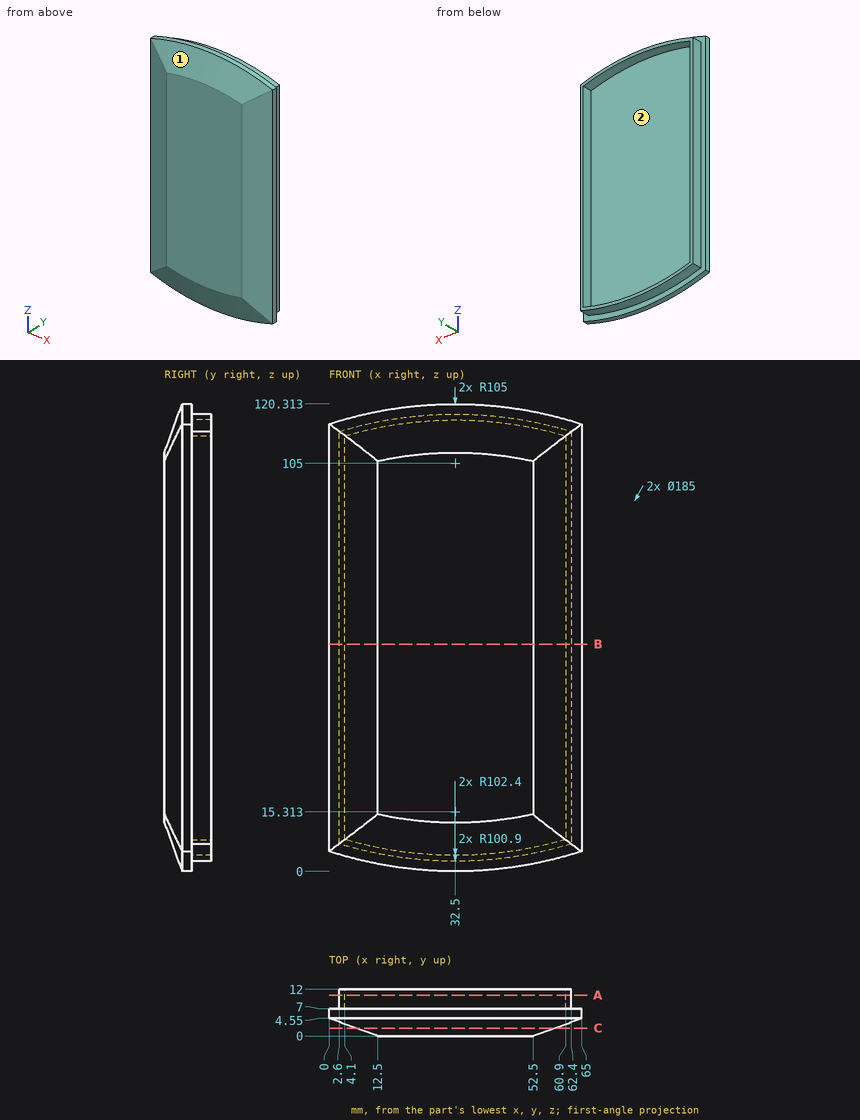
Job drawing, mm, ordinate dimensions from the low corner. One solid piece. A direction names the side the tool comes from. Round coordinates to 2 decimals unless told otherwise and drop trailing zeros. Loops run counter-clockwise (first coordinate to the right, second up) from the corner with the lowest first, then second, coordinate; pieces in that order, holes last.
Item 1: Drill centre lines: line 1 (X direction, y = 8, z = 104); line 2 (Z direction, x = 11.5, y = 10.5); line 3 (Z direction, x = 26.5, y = 8) (1 decimal). Where is each one in solid material? Low to high.
Item 2: Cut at C-C, the plane y = 2. Give the cut face in (x, z) (1 decimal), then the cut area to 3 significant figures.
Item 3: 3-axis set-ups, long thin cutter, end or side, ignore diameter. For the marked faces 1 and 2: which of +Z, -Z, +X, -X, +Y, -Y reach the whole face in a straight line?
Item 4: Cut at A-A, the plane y = 10.5. Give the cut face in (x, z).
Item 5: Drop flat-ended pins along their axis: P1, Ø6, axis at x = 50, y = 10.5, coming from the +Z side; P2, Ø2, axis at y = 4, z = 38.5, coming from the -X side; P3, Ø2.5, axis at y = 8.5, z = 43.5, coming from the -X side; P4, Ø5, axis at x = 52.5, y = 3, coming from the +Z side. Give the stop position or say it passes through.
Item 6: Cut at B-B, the plane z = 58.5. Give the cut face in (x, y).
A:
1. line 1: x = 2.6 to 4.1, 60.9 to 62.4
1. line 2: z = 4.78 to 6.31, 114 to 115.54
1. line 3: z = 2.8 to 4.3, 116 to 117.5
2. outline: (7, 10.4) arc R98 ccw to (58, 10.4) - (58, 109.9) arc R98 ccw to (7, 109.9) - close
2. area: 5,310 mm2
3. face 1: +Z, -Y
3. face 2: +Y
4. outline: (2.6, 7.06) arc R102.4 ccw to (62.4, 7.06) - (62.4, 113.25) arc R102.4 ccw to (2.6, 113.25) - close; hole (4.1, 8.18) arc R100.9 ccw to (60.9, 8.18) - (60.9, 112.13) arc R100.9 ccw to (4.1, 112.13) - close
5. P1: stops at z = 116.68
5. P2: stops at x = 0
5. P3: stops at x = 2.6
5. P4: stops at z = 118.75
6. outline: (0, 4.55) - (12.5, 0) - (52.5, 0) - (65, 4.55) - (65, 7) - (62.4, 7) - (62.4, 12) - (60.9, 12) - (60.9, 7) - (4.1, 7) - (4.1, 12) - (2.6, 12) - (2.6, 7) - (0, 7) - close
